Design review of the part shown in the three views and the two pictorial views. Dimensions are in mm from the part's minimum x, y and z. Coordinates: 2 decimals unless noted, no trailing zeros. Write each loop counter-clockwise with the first axis right and the second up, starting at its lowest first coordinate (ties: lowest second). Pieces come first, ordered by that corner, then holes. Notation, with made-up numbers: (80.25, 48) - (99.25, 48) arc R25 ccw to (99.25, 65) - close; hole circle Ø6 at (18, 9.5). An arc over 180 degrees is marked (long way). Return JSON: item names as keys, results as strings. Group by question number.
(1) For pin 1 Ø2.5 at (x, y) = (5, 29.5) entering from +Z, flat-tipped, find the tip position at first contact; note if it passes through.
(2) To check wall thickness, follow L1, parallel to Y at x = 5, z = 152; L2, parallel to X at y = 15.5, z = 152.75; L3, parallel to Z at x = 7.5, y = 13. State the ranges of each line that lie inside material, in increasing order. Write a range as from..to.
(3) We need section A-A on x = 5. State the section outline as (y, z) points, then the cut area to 3 significant figures.
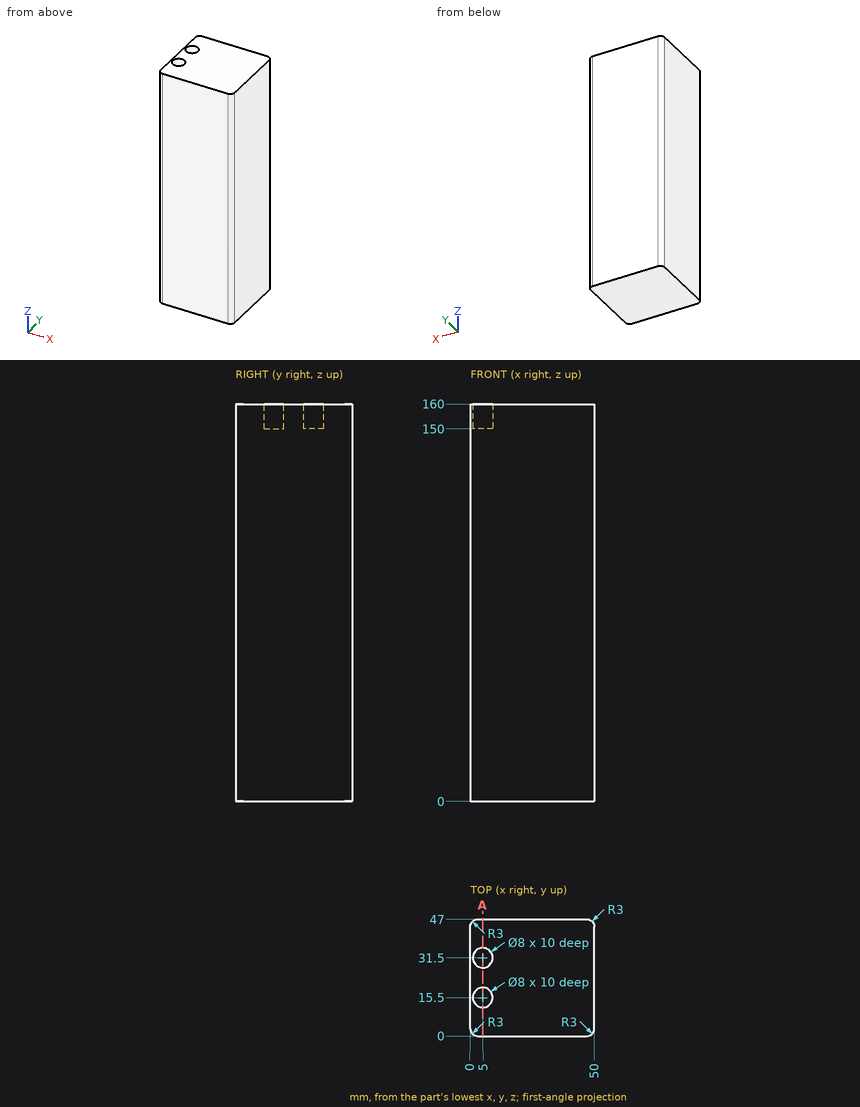
Ans:
{
 "1": {"pin 1": "z = 150"},
 "2": {"L1": "0..11.5, 19.5..27.5, 35.5..47", "L2": "0..1, 9..50", "L3": "0..150"},
 "3": {"outline": "(0, 0) - (47, 0) - (47, 160) - (35.5, 160) - (35.5, 150) - (27.5, 150) - (27.5, 160) - (19.5, 160) - (19.5, 150) - (11.5, 150) - (11.5, 160) - (0, 160) - close", "area": "7,360 mm²"}
}
